Geometry check sheet. Reference: the model listing, model coordinates, mm. Face numbers are marked on the shaded views. A direction names the side the tool comes from. Give positions to 0.01 mm unless a question says otherwise; leave off trailing zeros. Write each loop counter-clockwise with the first axis right and the second up, starting at its lowest first coordinate (ties: lowest second). Pieces come first, ordered by that corner, then holes.
(1) Cross-section at D-D (y = 108). Record the boundary of the cut face in (x, z), and give its area (3 significant figures).
(2) Thickness scan on line 1 along Z through (x, y) = (-25.5, 24); line 2 along X through (y, z) = (14, 0); line 3 along Y through (x, z) = (0, -10). Record the ranges inside material, lowest first.
(3) Cross-section at B-B (z = 0). Count the separate pieces of the cut face and the enclosed holes in it, and give its area (3 significant figures).
(4) Tool access check on the marked faces 1, 2, 3 and 4. Record the directions out of +Z, -Z, +X, -X, +Y, -Y that give a thin tool (end or side, any length) a straight path to the whole face; none if there is none.
(5) Cross-section at A-A (x = 0). Record the boundary of the cut face in (y, z).
(6) Cross-section at C-C (y = 141.5). Record the boundary of the cut face in (x, z).
(7) Depth check by flat-ended pin: P1, Ø2, axis at x = 12, y = 37, coming from the -Z side; P2, Ø6, axis at y = 114, z = 8.5, coming from the -X side; P3, Ø10, axis at x = -1, y = 95.5, coming from the +Z side. Enter the tip coordinate at first touch or a pass-through.
```python
from build123d import *

# Parameters (mm, degrees)
SKETCH_2_R               = 75
EXTRUDE_1_DEPTH          = 15
SKETCH_3_R               = 6
EXTRUDE_2_DEPTH          = 14
CUT_EXTRUDE_2_DEPTH      = 188.81639971
CUT_EXTRUDE_2_DEPTH_BACK = 188.81639971
SKETCH_4_W               = 12
SKETCH_4_H               = 150
SKETCH_5_R               = 40
CUT_EXTRUDE_3_DEPTH      = 7.5
CHAMFER_2_SIZE           = 5
RIB_21_REACH             = 189.816
SKETCH_8_WALL_W          = 468.456805058
SKETCH_8_WALL_H          = 10
PATTERN_CIRCULAR_3_COUNT = 6


with BuildPart() as part:
    # 草图2 → 凸台-拉伸1 (new body)
    with BuildSketch(Plane(origin=(0, 0, 0), x_dir=(1, 0, 0), z_dir=(0, 1, 0))):
        with Locations(Location((0, 0, 0), (0, 0, 270))):
            Circle(SKETCH_2_R)
    extrude(amount=EXTRUDE_1_DEPTH)

    # 草图3 → 凸台-拉伸2 (add, symmetric)
    with BuildSketch(Plane.XY):
        with BuildLine():
            Line((10, 145), (10, 130))
            Line((10, 130), (40, 15))
            Line((40, 15), (-40, 15))
            Line((-40, 15), (-10, 130))
            Line((-10, 130), (-10, 145))
            ThreePointArc((-10, 145), (0, 155), (10, 145))
        make_face()
        with Locations((0, 145)):
            Circle(SKETCH_3_R, mode=Mode.SUBTRACT)
    extrude(amount=EXTRUDE_2_DEPTH, both=True)

    # 草图4 → 切除-拉伸2 (cut, two sides: drawn at the far end of the back side and taken through both)
    with BuildSketch(Plane(origin=(0, 0, 0), x_dir=(0, 0, -1), z_dir=(1, 0, 0)).offset(-CUT_EXTRUDE_2_DEPTH_BACK)):
        with Locations((0, 90)):
            Rectangle(SKETCH_4_W, SKETCH_4_H)
    extrude(amount=CUT_EXTRUDE_2_DEPTH + CUT_EXTRUDE_2_DEPTH_BACK, mode=Mode.SUBTRACT)

    # 草图5 → 切除-拉伸3 (cut)
    with BuildSketch(Plane(origin=(0, 0, 0), x_dir=(1, 0, 0), z_dir=(0, 1, 0))):
        with Locations(Location((0, 0, 0), (0, 0, 270))):
            Circle(SKETCH_5_R)
    extrude(amount=CUT_EXTRUDE_3_DEPTH, mode=Mode.SUBTRACT)

    # 倒角2
    chamfer_2_edges = [part.edges().sort_by_distance(p)[0] for p in [
        (0, 15, -75),
    ]]
    chamfer(chamfer_2_edges, length=CHAMFER_2_SIZE)

    # 草图8 wall → 筋21 (add, up to next)
    with BuildSketch(Plane(origin=(0, 57.5, 30), x_dir=(0, -0.935875921829, 0.352329758806), z_dir=(0, -0.352329758806, -0.935875921829)), mode=Mode.PRIVATE) as rib_21_sk1:
        Rectangle(SKETCH_8_WALL_W, SKETCH_8_WALL_H)
    rib_21_tool1 = extrude(rib_21_sk1.sketch, amount=RIB_21_REACH, mode=Mode.PRIVATE) - part.part
    rib_21 = rib_21_tool1.solids().sort_by_distance((0, 57.5, 30))[0]
    add(rib_21)

    # 镜向1: 筋21 across plane
    add(rib_21.mirror(Plane.XY))

    # 草图24 → M8 六角头螺栓C级的柱形沉头孔7 (revolve, cut)
    with BuildSketch(Plane(origin=(-59.477689935, 15, 0), x_dir=(0, 0, 1), z_dir=(1, 0, 0))):
        Polygon((0, 0), (0, 15), (4.5, 15), (4.5, 0.5), (9, 0.5), (9, 0.020977491), (9.025, 0), align=None)
    m8_c_7 = revolve(axis=Axis((-59.477689935, 21.35, 0), (0, -1, 0)), mode=Mode.SUBTRACT)

    # 阵列(圆周)3: M8 六角头螺栓C级的柱形沉头孔7 ×6 about axis
    pattern_circular_3_axis = Axis((1.151424032, 0, 0), (0, 1, 0))
    for i in range(1, PATTERN_CIRCULAR_3_COUNT):
        add(m8_c_7.rotate(pattern_circular_3_axis, i * 360 / PATTERN_CIRCULAR_3_COUNT), mode=Mode.SUBTRACT)


solid = part.part
```
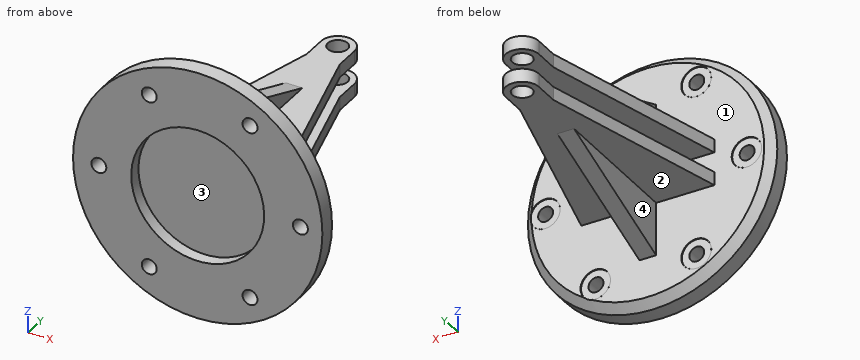
Reply:
1. outline: (-15.74, -14) - (15.74, -14) - (15.74, -6) - (-15.74, -6) - close; (-15.74, 6) - (15.74, 6) - (15.74, 14) - (-15.74, 14) - close
1. area: 504 mm2
2. line 1: z = -14 to -6, 6 to 14
2. line 2: x = -71 to -63.98, -54.98 to 57.28, 66.28 to 71
2. line 3: y = 7.5 to 139, 151 to 155
3. separate pieces: 3
3. enclosed holes: 0
3. area: 1,350 mm2
4. face 1: +Y
4. face 2: -Z, +Y
4. face 3: -Y
4. face 4: -Z, -X, +Y
5. outline: (0, -75) - (10, -75) - (15, -70) - (15, -46) - (100, -14) - (139, -14) - (139, -6) - (15, -6) - (15, 6) - (139, 6) - (139, 14) - (100, 14) - (15, 46) - (15, 70) - (10, 75) - (0, 75) - (0, 40) - (7.5, 40) - (7.5, -40) - (0, -40) - close; (151, -14) - (155, -14) - (155, -6) - (151, -6) - close; (151, 6) - (155, 6) - (155, 14) - (151, 14) - close
6. outline: (-10, -14) - (-4.87, -14) - (-4.87, -6) - (-10, -6) - close; (-10, 6) - (-4.87, 6) - (-4.87, 14) - (-10, 14) - close; (4.87, -14) - (10, -14) - (10, -6) - (4.87, -6) - close; (4.87, 6) - (10, 6) - (10, 14) - (4.87, 14) - close
7. P1: stops at z = -14
7. P2: stops at x = -14.96
7. P3: stops at z = 17.58
